from build123d import *

# Parameters (mm, degrees)
F0_W     = 101.6
F0_H     = 63.5
F1_DEPTH = 12.7
F2_R     = 6.35
F3_DEPTH = 12.701
F4_W     = 12.7
F4_H     = 38.1
F6_W     = 25.375047
F6_H     = 12.7


with BuildPart() as f1:
    # F0 (on Top) → F1 (new body)
    with BuildSketch(Plane.XY):
        with Locations((2.934791, 6.967624)):
            Rectangle(F0_W, F0_H)
    extrude(amount=F1_DEPTH)

    # F2 (on face) → F3 (cut, through all)
    with BuildSketch(Plane.XY.offset(12.7)):
        with Locations((-35.165209, 26.017624)):
            Circle(F2_R)
        with Locations((-35.165209, -12.082376)):
            Circle(F2_R)
        with Locations((41.034791, -12.082376)):
            Circle(F2_R)
        with Locations((41.034791, 26.017624)):
            Circle(F2_R)
    extrude(amount=-F3_DEPTH, mode=Mode.SUBTRACT)

    # F4 (on Front) → F5 (revolve)
    with BuildSketch(Plane.XZ):
        with Locations((-6.35, 31.75)):
            Rectangle(F4_W, F4_H)
    revolve(axis=Axis((0, 0, 31.75), (0, 0, -1)))

    # F6 (on Front) → F7 (revolve, cut)
    with BuildSketch(Plane.XZ):
        with Locations((-19.26654, 31.75)):
            Rectangle(F6_W, F6_H)
    revolve(axis=Axis((0, 0, 26.451318), (0, 0, 1)), mode=Mode.SUBTRACT)


solid = f1.part
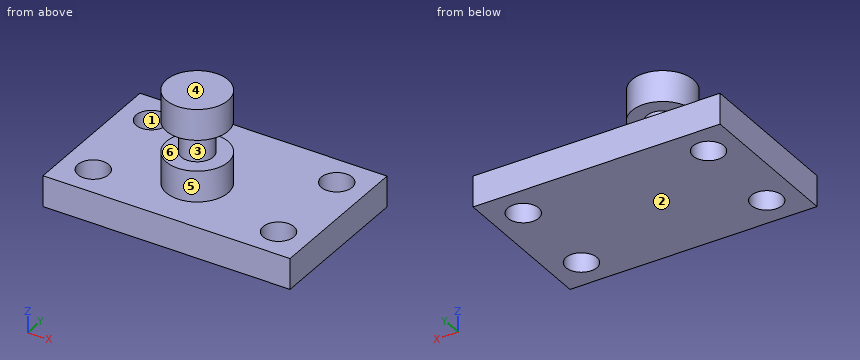
Design review of the part built by this model. Coordinates are the model's own, in mm. Face numbers are marked on the shaded views. A direction names the side the tool comes from. Give positions to 0.01 mm unless a question says otherwise; leave off trailing zeros. Loops run counter-clockwise (first coordinate to the right, second up) from the corner with the lowest first, then second, coordinate; pieces in that order, holes last. Notation, with made-up numbers: (81.5, 0.5) - (108.5, 0.5) arc R29 ccw to (108.5, 31.5) - close; hole circle Ø5 at (36, -37). An arc over 180 degrees is marked (long way). Write item = value, one per line.
1) Clearance check with flat-ended pins moving along their axes: pin 1 Ø4 at (y, z) = (2, 35.5) entering from +X; pin 2 Ø6 at (x, z) = (2, 16.5) entering from +Y; pin 3 Ø16.5 at (x, y) = (41.03, -12.08) entering from +Z. State where each tip first meets the part, or that it passes through.
Result sheet:
pin_1 = 6.58
pin_2 = 12.7
pin_3 = 12.7
2) To check wall thickness, follow line 1 (X direction, y = -12.5, z = 5.5); line 2 (Y direction, x = 43, z = 12.5); line 3 (Z direction, x = 2, y = 7.5). State the ranges of each line that lie inside material, in increasing order.
Result sheet:
line_1 = -47.87 to -41.5, -28.83 to 34.7, 47.37 to 53.73
line_2 = -24.78 to -18.12, -6.04 to 19.98, 32.06 to 38.72
line_3 = 0 to 25.4, 38.1 to 50.8
3) Tool access review of the marked faces 4, 5 and 6: name each direction out of +Z, -Z, +X, -X, +Y, -Y from which nothing blocks a thin tool from reaching the whole face with its end or side.
Result sheet:
face_4 = +Z, +X, -X, +Y, -Y
face_5 = +Z
face_6 = none
4) Take a section at C-C on y = -15. State the section outline as (x, z) points, and give its area (3 significant figures).
Result sheet:
outline = (-47.87, 0) - (-40.81, 0) - (-40.81, 12.7) - (-47.87, 12.7) - close; (-29.53, 0) - (35.39, 0) - (35.39, 12.7) - (-29.53, 12.7) - close; (46.67, 0) - (53.73, 0) - (53.73, 12.7) - (46.67, 12.7) - close
area = 1,000 mm2
5) Take a section at A-A on y = 0. State the section outline as (x, z) points.
Result sheet:
outline = (-47.87, 0) - (53.73, 0) - (53.73, 12.7) - (12.7, 12.7) - (12.7, 25.4) - (6.58, 25.4) - (6.58, 38.1) - (12.7, 38.1) - (12.7, 50.8) - (-12.7, 50.8) - (-12.7, 38.1) - (-6.58, 38.1) - (-6.58, 25.4) - (-12.7, 25.4) - (-12.7, 12.7) - (-47.87, 12.7) - close
6) Draft analysis for pull direction Z (two halves, no side actions). For the marked faces 1, 2 and 3, state which applies: +Z half, -Z half, draft (parallel to the pull), parting line (faces both ways), or undercut.
Result sheet:
face_1 = draft
face_2 = -Z half
face_3 = undercut
7) Take a section at D-D on x = 0. State the section outline as (y, z) points.
Result sheet:
outline = (-24.78, 0) - (38.72, 0) - (38.72, 12.7) - (12.7, 12.7) - (12.7, 25.4) - (6.58, 25.4) - (6.58, 38.1) - (12.7, 38.1) - (12.7, 50.8) - (-12.7, 50.8) - (-12.7, 38.1) - (-6.58, 38.1) - (-6.58, 25.4) - (-12.7, 25.4) - (-12.7, 12.7) - (-24.78, 12.7) - close
8) Take a section at B-B on x = 38.5. State the section outline as (y, z) points.
Result sheet:
outline = (-24.78, 0) - (-17.9, 0) - (-17.9, 12.7) - (-24.78, 12.7) - close; (-6.26, 0) - (20.2, 0) - (20.2, 12.7) - (-6.26, 12.7) - close; (31.84, 0) - (38.72, 0) - (38.72, 12.7) - (31.84, 12.7) - close
